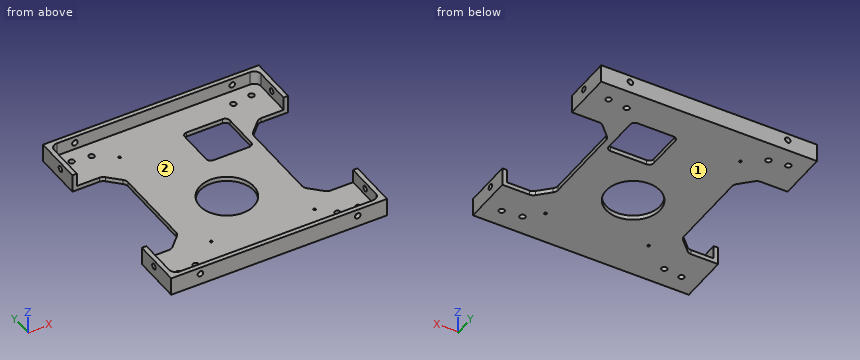
```python
from build123d import *

# Parameters (mm, degrees)
SKETCH1_W                      = 96
SKETCH1_H                      = 96
BOSS_EXTRUDE1_DEPTH            = 8
SKETCH2_W                      = 92
SKETCH2_H                      = 92
COMPONENT_PLATFORM_DEPTH       = 6
CABLE_SLOTS_DEPTH              = 6
INNER_CORNER_FILLETS_R         = 3
M3X0_5_TAPPED_HOLE1_AT_2_COUNT = 2
M3X0_5_TAPPED_HOLE1_AT_2_PITCH = 70
M3X0_5_TAPPED_HOLE2_AT_2_COUNT = 2
M3X0_5_TAPPED_HOLE2_AT_2_PITCH = 70
M1_4X0_3_TAPPED_HOLE1_D        = 1.1
M1_4X0_3_TAPPED_HOLE1_DEPTH    = 3.7
M1_4X0_3_TAPPED_HOLE1_TIP      = 0.33047334
SKETCH29_R                     = 12
HDD_EXTRUSION_CUTOUT_DEPTH     = 10
HDD_EXTRUSION_CUTOUT_2_DEPTH   = 10
M3X0_5_TAPPED_HOLE3_D          = 2.5
M3X0_5_TAPPED_HOLE3_DEPTH      = 10
M3X0_5_TAPPED_HOLE3_TIP        = 0.751075774
M3X0_5_TAPPED_HOLE4_D          = 2.5


with BuildPart() as part:
    # Sketch1 → Boss-Extrude1 (new body)
    with BuildSketch(Plane.XY):
        Rectangle(SKETCH1_W, SKETCH1_H)
    extrude(amount=BOSS_EXTRUDE1_DEPTH)

    # Sketch2 → Component Platform (cut)
    with BuildSketch(Plane.XY.offset(8)):
        Rectangle(SKETCH2_W, SKETCH2_H)
    extrude(amount=-COMPONENT_PLATFORM_DEPTH, mode=Mode.SUBTRACT)

    # Sketch3 → Cable Slots (cut, symmetric)
    with BuildSketch(Plane.XY.offset(2)):
        with BuildLine():
            Line((-33.878679656, -25.121320344), (-28.878679656, -20.121320344))
            ThreePointArc((-28.878679656, -20.121320344), (-28.228361402, -19.148050297), (-28, -18))
            Line((-28, -18), (-28, 18))
            ThreePointArc((-28, 18), (-28.228361402, 19.148050297), (-28.878679656, 20.121320344))
            Line((-28.878679656, 20.121320344), (-33.878679656, 25.121320344))
            ThreePointArc((-33.878679656, 25.121320344), (-34.851949703, 25.771638598), (-36, 26))
            Line((-36, 26), (-48, 26))
            Line((-48, 26), (-48, -26))
            Line((-48, -26), (-36, -26))
            ThreePointArc((-36, -26), (-34.851949703, -25.771638598), (-33.878679656, -25.121320344))
        make_face()
        with BuildLine():
            Line((48, -26), (48, 26))
            Line((48, 26), (36, 26))
            ThreePointArc((36, 26), (34.851949703, 25.771638598), (33.878679656, 25.121320344))
            Line((33.878679656, 25.121320344), (28.878679656, 20.121320344))
            ThreePointArc((28.878679656, 20.121320344), (28.228361402, 19.148050297), (28, 18))
            Line((28, 18), (28, -18))
            ThreePointArc((28, -18), (28.228361402, -19.148050297), (28.878679656, -20.121320344))
            Line((28.878679656, -20.121320344), (33.878679656, -25.121320344))
            ThreePointArc((33.878679656, -25.121320344), (34.851949703, -25.771638598), (36, -26))
            Line((36, -26), (48, -26))
        make_face()
    extrude(amount=CABLE_SLOTS_DEPTH, both=True, mode=Mode.SUBTRACT)

    # Inner Corner Fillets
    inner_corner_fillets_edges = [part.edges().sort_by_distance(p)[0] for p in [
        (-46, -46, 5),
        (-46, 46, 5),
        (46, 46, 5),
        (46, -46, 5),
    ]]
    fillet(inner_corner_fillets_edges, radius=INNER_CORNER_FILLETS_R)

    # Sketch14 → M3x0.5 Tapped Hole1 (revolve, cut)
    with BuildSketch(Plane(origin=(48, -35, 5), x_dir=(0, 0, -1), z_dir=(0, 1, 0))):
        Polygon((0, 0), (0, 10.751075774), (1.25, 10), (1.25, 0), align=None)
    m3x0_5_tapped_hole1 = revolve(axis=Axis((54.35, -35, 5), (-1, 0, 0)), mode=Mode.SUBTRACT)

    # M3x0.5 Tapped Hole1 at 2: M3x0.5 Tapped Hole1 ×2
    with Locations(*[(0, i * M3X0_5_TAPPED_HOLE1_AT_2_PITCH, 0) for i in range(1, M3X0_5_TAPPED_HOLE1_AT_2_COUNT)]):
        add(m3x0_5_tapped_hole1, mode=Mode.SUBTRACT)

    # Sketch16 → M3x0.5 Tapped Hole2 (revolve, cut)
    with BuildSketch(Plane(origin=(35, 48, 5), x_dir=(0, 0, 1), z_dir=(1, 0, 0))):
        Polygon((0, 0), (0, 10.751075774), (1.25, 10), (1.25, 0), align=None)
    m3x0_5_tapped_hole2 = revolve(axis=Axis((35, 54.35, 5), (0, -1, 0)), mode=Mode.SUBTRACT)

    # M3x0.5 Tapped Hole2 at 2: M3x0.5 Tapped Hole2 ×2
    with Locations(*[(-i * M3X0_5_TAPPED_HOLE2_AT_2_PITCH, 0, 0) for i in range(1, M3X0_5_TAPPED_HOLE2_AT_2_COUNT)]):
        add(m3x0_5_tapped_hole2, mode=Mode.SUBTRACT)

    # Mirror1: M3x0.5 Tapped Hole1 across plane
    add(m3x0_5_tapped_hole1.mirror(Plane(origin=(0, 0, 0), x_dir=(0, 0, 1), z_dir=(1, 0, 0))), mode=Mode.SUBTRACT)

    # Mirror1 copy 1 sketch → Mirror1 copy 1 (revolve, cut)
    with BuildSketch(Plane(origin=(-48, 35, 5), x_dir=(0, 0, -1), z_dir=(0, 1, 0))):
        Polygon((0, 0), (0, -10.751075774), (1.25, -10), (1.25, 0), align=None)
    revolve(axis=Axis((-54.35, 35, 5), (-1, 0, 0)), mode=Mode.SUBTRACT)

    # Mirror2: M3x0.5 Tapped Hole2 across plane
    add(m3x0_5_tapped_hole2.mirror(Plane(origin=(0, 0, 0), x_dir=(0, 0, 1), z_dir=(0, -1, 0))), mode=Mode.SUBTRACT)

    # Mirror2 copy 1 sketch → Mirror2 copy 1 (revolve, cut)
    with BuildSketch(Plane(origin=(-35, -48, 5), x_dir=(0, 0, 1), z_dir=(1, 0, 0))):
        Polygon((0, 0), (0, -10.751075774), (1.25, -10), (1.25, 0), align=None)
    revolve(axis=Axis((-35, -54.35, 5), (0, -1, 0)), mode=Mode.SUBTRACT)

    # M1.4x0.3 Tapped Hole1
    with Locations(Plane.XY.offset(2)):
        with Locations((-19.31998517, -29.75), (24.78001483, -32.85), (-22.91998517, 32.85)):
            Hole(M1_4X0_3_TAPPED_HOLE1_D / 2, depth=M1_4X0_3_TAPPED_HOLE1_DEPTH)
            with Locations((0, 0, -(M1_4X0_3_TAPPED_HOLE1_DEPTH + M1_4X0_3_TAPPED_HOLE1_TIP / 2))):  # 118° drill point
                Cone(0, M1_4X0_3_TAPPED_HOLE1_D / 2, M1_4X0_3_TAPPED_HOLE1_TIP, mode=Mode.SUBTRACT)

    # Sketch29 → HDD Extrusion Cutout (cut)
    with BuildSketch(Plane(origin=(0, 0, 0), x_dir=(-1, 0, 0), z_dir=(0, 0, -1))):
        with Locations((-0.08192631, -8.74785827)):
            Circle(SKETCH29_R)
    extrude(amount=-HDD_EXTRUSION_CUTOUT_DEPTH, mode=Mode.SUBTRACT)

    # Sketch9 → HDD Extrusion Cutout 2 (cut)
    with BuildSketch(Plane.XY.offset(2)):
        with BuildLine():
            Line((25, 31), (25, 15))
            ThreePointArc((25, 15), (24.414213562, 13.585786438), (23, 13))
            Line((23, 13), (7, 13))
            ThreePointArc((7, 13), (5.585786438, 13.585786438), (5, 15))
            Line((5, 15), (5, 31))
            ThreePointArc((5, 31), (5.585786438, 32.414213562), (7, 33))
            Line((7, 33), (23, 33))
            ThreePointArc((23, 33), (24.414213562, 32.414213562), (25, 31))
        make_face()
    extrude(amount=-HDD_EXTRUSION_CUTOUT_2_DEPTH, mode=Mode.SUBTRACT)

    # M3x0.5 Tapped Hole3
    with Locations(Plane.XY.offset(2)):
        with Locations((-31.790998517, -39.06), (31.29001483, -39.06), (31.29001483, 38.94), (-31.790998517, 38.94)):
            Hole(M3X0_5_TAPPED_HOLE3_D / 2, depth=M3X0_5_TAPPED_HOLE3_DEPTH)
            with Locations((0, 0, -(M3X0_5_TAPPED_HOLE3_DEPTH + M3X0_5_TAPPED_HOLE3_TIP / 2))):  # 118° drill point
                Cone(0, M3X0_5_TAPPED_HOLE3_D / 2, M3X0_5_TAPPED_HOLE3_TIP, mode=Mode.SUBTRACT)

    # M3x0.5 Tapped Hole4 (through all)
    with Locations(Plane.XY.offset(2)):
        with Locations((40, -40), (-40, -40), (-40, 40), (40, 40)):
            Hole(M3X0_5_TAPPED_HOLE4_D / 2)


solid = part.part
```
The listing builds one solid part. Answer for the finished solid, in the listing's coordinates (mm). Face numbers are marked on the shaded views. Round coordinates to 2 decimals unless told otherwise and drop trailing zeros. Loops run counter-clockwise (first coordinate to the right, second up) from the corner with the lowest first, then second, coordinate; pieces in that order, holes last. Notation, with made-up numbers: (-26.5, 72) - (16.5, 72) arc R27 cw to (16.5, 111) - close; hole circle Ø9 at (-25, 69.25). An arc over 180 degrees is marked (long way). Use one line per item in the form item = value. Start each with the question number.
1. The part is cut by section D-D on y = -28. Determine the outline of the cut face in (x, z), then the cut area to 3 significant figures.
2. The part is cut by section B-B on y = 2. Determine the outline of the cut face in (x, z).
3. The part is cut by section A-A on x = -40. Determine the outline of the cut face in (y, z).
4. Given pin 1 Ø5 at (x, y) = (-31, 23) entering from -Z; pin 2 Ø1 at (y, z) = (6, 1) entering from +X; pin 3 Ø5 at (x, y) = (-0.5, -32.5) entering from +Z; pin 4 Ø0.6 at (y, z) = (20, 1) entering from -X, each flat-ended and moving along its own axis, determine where each tip first touches the part or whether it passes through.
5. The part is cut by section C-C on x = -1. Determine the outline of the cut face in (y, z), then the cut area to 3 significant figures.
6. For a pull along Y with two mould halves and no side action, classify the marked faces 1 and 2 as pulls with the +Y half, pulls with the -Y half, needs draft (parallel to the pull), parting line crosses it, or undercut.
7. Consider line 1 (X direction, y = -46.8, z = 5); line 2 (Y direction, x = -46.75, z = 5); line 3 (Y direction, x = -40, z = 1.35). Determine where each line is inside the solid, lowest interval first. Write a range as [from, to].
Geometry check:
q1.outline = (-48, 0) - (48, 0) - (48, 8) - (46, 8) - (46, 2) - (-46, 2) - (-46, 8) - (-48, 8) - close
q1.area = 216 mm^2
q2.outline = (-28, 0) - (-5.26, 0) - (-5.26, 2) - (-28, 2) - close; (5.42, 0) - (28, 0) - (28, 2) - (5.42, 2) - close
q3.outline = (-48, 0) - (-41.25, 0) - (-41.25, 2) - (-46, 2) - (-46, 8) - (-48, 8) - close; (-38.75, 0) - (-26, 0) - (-26, 2) - (-38.75, 2) - close; (26, 0) - (38.75, 0) - (38.75, 2) - (26, 2) - close; (41.25, 0) - (48, 0) - (48, 8) - (46, 8) - (46, 2) - (41.25, 2) - close
q4.pin_1 = 0
q4.pin_2 = 28
q4.pin_3 = 2
q4.pin_4 = -29.06
q5.outline = (-48, 0) - (-20.7, 0) - (-20.7, 2) - (-46, 2) - (-46, 8) - (-48, 8) - close; (3.2, 0) - (48, 0) - (48, 8) - (46, 8) - (46, 2) - (3.2, 2) - close
q5.area = 168 mm^2
q6.face_1 = needs draft
q6.face_2 = undercut
q7.line_1 = [-48, -36.25], [-33.75, 33.75], [36.25, 48]
q7.line_2 = [-48, -36.25], [-33.75, -26], [26, 33.75], [36.25, 48]
q7.line_3 = [-48, -41.25], [-38.75, -26], [26, 38.75], [41.25, 48]
